Input: part model. Units: mm. Frame: model coordinates. A direction names the side the tool comes from. Round coordinates to 2 decimals unless told otherwise and drop trailing zeros. Write each loop counter-clockwise with the first axis right and the second up, starting at its lowest first coordinate (ties: lowest second). Pieces come first, ordered by that corner, then holes. Notation, with made-up numbers: (21.5, 87.5) - (37.5, 87.5) arc R14 ccw to (37.5, 97.5) - close; hole circle Ø2 at (88.25, 22.5). An arc over 180 degrees is marked (long way). One line per item, written item: value. Start each with the question number.
```python
from build123d import *

# Parameters (mm, degrees)
SFAZOWANIE1_SIZE               = 0.5
ZAOKR_GLENIE1_R                = 0.5
OTWORY_USTALAJ_CE_8_0MM1_D     = 7.5
OTWORY_USTALAJ_CE_8_0MM1_DEPTH = 2
OTWORY_USTALAJ_CE_8_0MM1_TIP   = 2.253227321
ZAOKR_GLENIE2_R                = 1
SFAZOWANIE2_SIZE               = 0.5
WYTNIJ_WYCI_GNI_CIE1_DEPTH     = 3


with BuildPart() as part:
    # Szkic1 → Obrót1 (revolve)
    with BuildSketch(Plane.XY, mode=Mode.PRIVATE) as obr_t1_sk:
        Polygon((0, 0), (0, 2.35), (16, 2.35), (16, 10), (19, 10), (19, 5), (29, 5), (29, 4.6), (30.1, 4.6), (30.1, 5), (32, 5), (32, 0), align=None)
    revolve(obr_t1_sk.sketch.rotate(Axis((0, 0, 0), (-1, 0, 0)), 90), axis=Axis((0, 0, 0), (-1, 0, 0)))

    # Sfazowanie1
    sfazowanie1_edges = [part.edges().sort_by_distance(p)[0] for p in [
        (0, 0, 2.35),
    ]]
    chamfer(sfazowanie1_edges, length=SFAZOWANIE1_SIZE)

    # Zaokrąglenie1
    zaokr_glenie1_edges = [part.edges().sort_by_distance(p)[0] for p in [
        (16, 0, 2.35),
    ]]
    fillet(zaokr_glenie1_edges, radius=ZAOKR_GLENIE1_R)

    # Otwory ustalające Ø8.0mm1
    with Locations(Plane(origin=(32, 0, 0), x_dir=(0, 0, -1), z_dir=(1, 0, 0))):
        with Locations((0, 0)):
            Hole(OTWORY_USTALAJ_CE_8_0MM1_D / 2, depth=OTWORY_USTALAJ_CE_8_0MM1_DEPTH)
            with Locations((0, 0, -(OTWORY_USTALAJ_CE_8_0MM1_DEPTH + OTWORY_USTALAJ_CE_8_0MM1_TIP / 2))):  # 118° drill point
                Cone(0, OTWORY_USTALAJ_CE_8_0MM1_D / 2, OTWORY_USTALAJ_CE_8_0MM1_TIP, mode=Mode.SUBTRACT)

    # Zaokrąglenie2
    zaokr_glenie2_edges = [part.edges().sort_by_distance(p)[0] for p in [
        (19, 0, 5),
    ]]
    fillet(zaokr_glenie2_edges, radius=ZAOKR_GLENIE2_R)

    # Sfazowanie2
    sfazowanie2_edges = [part.edges().sort_by_distance(p)[0] for p in [
        (32, 0, 5),
    ]]
    chamfer(sfazowanie2_edges, length=SFAZOWANIE2_SIZE)

    # Szkic5 → Wytnij-wyciągnięcie1 (cut)
    with BuildSketch(Plane(origin=(19, 0, 0), x_dir=(0, 0, -1), z_dir=(1, 0, 0))):
        with BuildLine():
            Line((7.5, 6.614378278), (7.5, -6.614378278))
            ThreePointArc((7.5, -6.614378278), (9.354143467, -3.535533906), (10, 0))
            ThreePointArc((10, 0), (9.354143467, 3.535533906), (7.5, 6.614378278))
        make_face()
        with BuildLine():
            ThreePointArc((-7.5, 6.614378278), (-10, 0), (-7.5, -6.614378278))
            Line((-7.5, -6.614378278), (-7.5, 6.614378278))
        make_face()
    extrude(amount=-WYTNIJ_WYCI_GNI_CIE1_DEPTH, mode=Mode.SUBTRACT)


solid = part.part
```
Q1. Cut plane B-B, the plane x = 10.5. Output: boundary loops of the cut face in (y, z), and give its area (3 significant figures).
Q2. Pull-direction query (X, two-part tool) for faces 1 (the flat face through (32, -4, 1)), 2 (the flat face through (0, 0, 0)), 3 (the cylindrical face through (31, 0, 5)), 4 (the cylindrical face through (29.56, 2.8, 3.65)); classes: pulls with the +X half, pulls with the -X half, needs draft (parallel to the pull), parting line crosses it, or undercut.
Q3. Cut plane A-A, the plane x = 17.5. Output: boundary loops of the cut face in (y, z).
Q4. Access query for faces 5 (the cylindrical face through (18, 10, 0)), 6 (the flat face through (19, -7, 0)), 7 (the cylindrical face through (8.105, 2.294, 0.509)). Directions: +Z, -Z, +X, -X, +Y, -Y. A direction counts if a zero-diameter tool reaches every point of the face in a straight line with its end or side. Return the directions, or none.
Q5. Material intervals for probe 1 along Y at (x, z) = (31, 0); probe 2 along X at (y, z) = (-6, 0.75); probe 3 along X at (y, z) = (-1.5, 1.5), sorted ascending. Write a range as from..to.
Q6. Contact query for flat-ended pins moving along their axis: pin 1 Ø5 at (x, y) = (3.5, 2) entering from -Z; pin 2 Ø4.5 at (y, z) = (-0.5, -0.5) entering from +X; pin 3 Ø2 at (y, z) = (2.5, -1) entering from +X. Output: stop coordinate, or through.
A:
1. outline: circle Ø4.7 at (0, 0)
1. area: 17.3 mm²
2. face 1: pulls with the +X half
2. face 2: pulls with the -X half
2. face 3: needs draft
2. face 4: undercut
3. outline: (-6.61, -7.5) - (6.61, -7.5) arc R10 ccw to (6.61, 7.5) - (-6.61, 7.5) arc R10 ccw to start
4. face 5: +X, -X, +Y
4. face 6: +X
4. face 7: -X
5. probe 1: y = -5..-3.75, 3.75..5
5. probe 2: x = 16..19
5. probe 3: x = 0.27..29.02
6. pin 1: stops at z = -2.35
6. pin 2: stops at x = 29.52
6. pin 3: stops at x = 29.97
